```python
from build123d import *

# Parameters (mm, degrees)
EXTRUDE_1_DEPTH     = 10
CUT_EXTRUDE_5_REACH = 34.402
SKETCH_7_R          = 1.5
SKETCH_8_W          = 15.3
SKETCH_8_H          = 15.3
CUT_EXTRUDE_6_DEPTH = 10
SKETCH_11_R         = 1.5
CUT_EXTRUDE_8_DEPTH = 37.769552622


with BuildPart() as part:
    # 草图1 → 凸台-拉伸1 (new body)
    with BuildSketch(Plane.XY):
        Polygon((-26, 4.55), (-26, 1.55), (-3, 1.55), (-3, -1.55), (-26, -1.55), (-26, -4.55), (-7, -4.55), (0, -12), (26, -12), (26, 12), (0, 12), (-7, 4.55), align=None)
    extrude(amount=EXTRUDE_1_DEPTH)

    # 切除-拉伸5: up to this face of the body (flat: up to its plane)
    cut_extrude_5_end = Plane(part.part.faces().sort_by_distance((-16.5, -4.55, 5))[0])
    # 草图7 → 切除-拉伸5 (cut, up to the picked face)
    with BuildSketch(Plane(origin=(0, 4.55, 0), x_dir=(1, 0, 0), z_dir=(0, 1, 0)), mode=Mode.PRIVATE) as cut_extrude_5_sk1:
        with Locations(Location((-21, -5, 0), (0, 0, 270))):
            Circle(SKETCH_7_R)
    cut_extrude_5_tool1 = split(extrude(cut_extrude_5_sk1.sketch, amount=-CUT_EXTRUDE_5_REACH, mode=Mode.PRIVATE), bisect_by=cut_extrude_5_end, keep=Keep.BOTH, mode=Mode.PRIVATE)
    # 草图7 → 切除-拉伸5 (cut, up to the picked face)
    with BuildSketch(Plane(origin=(0, 4.55, 0), x_dir=(1, 0, 0), z_dir=(0, 1, 0)), mode=Mode.PRIVATE) as cut_extrude_5_sk2:
        with Locations(Location((-9, -5, 0), (0, 0, 270))):
            Circle(SKETCH_7_R)
    cut_extrude_5_tool2 = split(extrude(cut_extrude_5_sk2.sketch, amount=-CUT_EXTRUDE_5_REACH, mode=Mode.PRIVATE), bisect_by=cut_extrude_5_end, keep=Keep.BOTH, mode=Mode.PRIVATE)
    add(cut_extrude_5_tool1.solids().sort_by(Axis((-21, 4.55, 5), (0, -1, 0)))[0], mode=Mode.SUBTRACT)
    add(cut_extrude_5_tool2.solids().sort_by(Axis((-9, 4.55, 5), (0, -1, 0)))[0], mode=Mode.SUBTRACT)

    # 草图8 → 切除-拉伸6 (cut)
    with BuildSketch(Plane(origin=(0, 0, 0), x_dir=(-1, 0, 0), z_dir=(0, 0, -1))):
        with Locations((-18.35, 0.05)):
            Rectangle(SKETCH_8_W, SKETCH_8_H)
    extrude(amount=-CUT_EXTRUDE_6_DEPTH, mode=Mode.SUBTRACT)

    # 草图11 → 切除-拉伸8 (cut, through all)
    with BuildSketch(Plane.XZ.offset(12)):
        with Locations((20, 5)):
            Circle(SKETCH_11_R)
    extrude(amount=-CUT_EXTRUDE_8_DEPTH, mode=Mode.SUBTRACT)


solid = part.part
```
Can you work these out from the model? Positions are in its coordinate system, mm. A direction names the side the tool comes from. Round coordinates to 2 decimals unless told otherwise and drop trailing zeros. Loops run counter-clockwise (first coordinate to the right, second up) from the corner with the lowest first, then second, coordinate; pieces in that order, holes last. Notation, with made-up numbers: (25.5, 39.25) -> (44.5, 39.25) arc R14 cw to (44.5, 60.25) -> close; hole circle Ø10 at (72.5, -2). An arc over 180 degrees is marked (long way). One line per item, written item: value. Start each with the question number.
1. If we section it at B-B, the plane z = 1.5: Write out the boundary of the cut face in (x, y).
2. If we section it at C-C, the plane y = 8.5: Write out the boundary of the cut face in (x, z), then the cut area to 3 significant figures.
3. For faces 1 (the flat face through (-14, -1.55, 5)), 2 (the flat face through (-17, -4.55, 5)), 3 (the flat face through (18, 7.7, 5)), 4 (the flat face through (-16, 4.55, 5)), which set-ups out of +Z, -Z, +X, -X, +Y, -Y let a thin tool reach every point of the face, with its end or its side?
4. If we section it at D-D, the plane x = 19: Write out the boundary of the cut face in (y, z), then the cut area to 3 significant figures.
5. If I drill on probe 1 along X at (y, z) = (3.45, 5); probe 2 along Y at (x, z) = (18, 6); probe 3 along Y at (x, z) = (-8, 7.5), over which ranges is the centre line in solid material (lowest first)?
6. For pin 1 (3 mm diameter, centred on x = -17.5, z = 7.5, fed in from +Y); pin 2 (6 mm diameter, centred on y = -5.5, z = 6.5, fed in from -X); pin 3 (3.5 mm diameter, centred on x = -21, z = 5, fed in from -Y); pin 4 (1.5 mm diameter, centred on y = 9.5, z = 5, fed in from -X), each with a flat end and sliding along its axis, tell me the tip position at first contact or that it passes through.
7. If we section it at A-A, the plane x = -17: Write out the boundary of the cut face in (y, z), then the cut area to 3 significant figures.
8. If we mould it in two halves opening along Z, with no side actions, what happens to faces 5 (the flat face through (5, 0, 10)), 6 (the cylindrical face through (18.5, -9.83, 5.07)), 7 (the flat face through (-15, 1.55, 5)), 8 (the cylindrical face through (-19.735, -3.029, 5.806))? For each: pulls with the +Z half, pulls with the -Z half, needs draft (parallel to the pull), parting line crosses it, or undercut.
Calculated:
1. outline: (-26, -4.55) -> (-7, -4.55) -> (0, -12) -> (26, -12) -> (26, -7.6) -> (10.7, -7.6) -> (10.7, 7.7) -> (26, 7.7) -> (26, 12) -> (0, 12) -> (-7, 4.55) -> (-26, 4.55) -> (-26, 1.55) -> (-3, 1.55) -> (-3, -1.55) -> (-26, -1.55) -> close
2. outline: (-3.29, 0) -> (26, 0) -> (26, 10) -> (-3.29, 10) -> close; hole circle Ø3 at (20, 5)
2. area: 286 mm²
3. face 1: +Z, -Z, -X
3. face 2: +Z, -Z, -X, -Y
3. face 3: +Z, -Z, +X
3. face 4: +Z, -Z, -X, +Y
4. outline: (-12, 0) -> (-7.6, 0) -> (-7.6, 3.88) -> (-12, 3.88) -> close; (-12, 6.12) -> (-7.6, 6.12) -> (-7.6, 10) -> (-12, 10) -> close; (7.7, 0) -> (12, 0) -> (12, 3.88) -> (7.7, 3.88) -> close; (7.7, 6.12) -> (12, 6.12) -> (12, 10) -> (7.7, 10) -> close
4. area: 67.5 mm²
5. probe 1: x = -26 to -22.5, -19.5 to -10.5, -7.5 to 10.7
5. probe 2: y = -12 to -7.6, 7.7 to 12
5. probe 3: y = -4.55 to -1.55, 1.55 to 4.55
6. pin 1: stops at y = 4.55
6. pin 2: stops at x = -26
6. pin 3: stops at y = -4.55
6. pin 4: stops at x = -3.05
7. outline: (-4.55, 0) -> (-1.55, 0) -> (-1.55, 10) -> (-4.55, 10) -> close; (1.55, 0) -> (4.55, 0) -> (4.55, 10) -> (1.55, 10) -> close
7. area: 60.0 mm²
8. face 5: pulls with the +Z half
8. face 6: undercut
8. face 7: needs draft
8. face 8: undercut
